```python
from build123d import *

# Parameters (mm, degrees)
SKETCH_1_R               = 2.6
EXTRUDE_1_DEPTH          = 5
EXTRUDE_2_DEPTH          = 3.5
PATTERN_CIRCULAR_4_COUNT = 3


with BuildPart() as part:
    # 草图1 → 凸台-拉伸1 (new body)
    with BuildSketch(Plane(origin=(0, 0, 0), x_dir=(1, 0, 0), z_dir=(0, 1, 0))):
        with BuildLine():
            Line((-4.913295992, -4.857418706), (-3.181245185, -3.857418706))
            ThreePointArc((-3.181245185, -3.857418706), (0, -5), (3.181245185, -3.857418706))
            Line((3.181245185, -3.857418706), (4.913295992, -4.857418706))
            Line((4.913295992, -4.857418706), (6.663295992, -1.826329793))
            Line((6.663295992, -1.826329793), (4.931245185, -0.826329793))
            ThreePointArc((4.931245185, -0.826329793), (4.330127019, 2.5), (1.75, 4.683748499))
            Line((1.75, 4.683748499), (1.75, 6.683748499))
            Line((1.75, 6.683748499), (-1.75, 6.683748499))
            Line((-1.75, 6.683748499), (-1.75, 4.683748499))
            ThreePointArc((-1.75, 4.683748499), (-4.330127019, 2.5), (-4.931245185, -0.826329793))
            Line((-4.931245185, -0.826329793), (-6.663295992, -1.826329793))
            Line((-6.663295992, -1.826329793), (-4.913295992, -4.857418706))
        make_face()
        with Locations(Location((0, 0, 0), (0, 0, 270))):
            Circle(SKETCH_1_R, mode=Mode.SUBTRACT)
    extrude(amount=EXTRUDE_1_DEPTH)

    # 草图2 → 凸台-拉伸2 (add)
    with BuildSketch(Plane(origin=(0.875, 0, 1.515544457), x_dir=(0.8660254037844383, 0, -0.5000000000000009), z_dir=(0.5000000000000008, 0, 0.8660254037844382))):
        Polygon((-4.683748499, 5), (-9.731723247, 13.632378058), (-11.731723247, 12.462833649), (-6.683748499, 3.830455591), align=None)
    extrude(amount=-EXTRUDE_2_DEPTH)


with BuildPart() as pattern_circular_4_1:
    # 阵列(圆周)4: pattern copy
    add(part.part.rotate(Axis((0, 0, 0), (0, 1, 0)), 1 * 360 / PATTERN_CIRCULAR_4_COUNT))


with BuildPart() as pattern_circular_4_2:
    # 阵列(圆周)4: pattern copy
    add(part.part.rotate(Axis((0, 0, 0), (0, 1, 0)), 2 * 360 / PATTERN_CIRCULAR_4_COUNT))


with BuildPart() as pattern_circular_4_1_1:
    add(pattern_circular_4_1.part)

    # Combine 1: read off the stored shape, not the designer's step
    # Combine 1: union 阵列(圆周)4_2, part
    add(pattern_circular_4_2.part)
    add(part.part)


solid = pattern_circular_4_1_1.part
```
Read the model definition and answer for the solid it produces. Units are mm, in the model's axes. A direction names the side the tool comes from. Give positions to 0.01 mm unless a question says otherwise; leave off trailing zeros. Order: outer loops, then holes, each group sorted by start corner. A loop starts at its lowest first (then second) coordinate and runs counter-clockwise, first axis right, second up.
(1) Find section D-D (z = -2). Give the vertices of the cut face in (x, y), plus the area to 3 significant figures.
(2) Find section A-A (x = 0). Give the vertices of the cut face in (y, z), plus the area to 3 significant figures.
(3) Given pin 1 (0.6 mm diameter, centred on y = 1.5, z = -5.5, fed in from -X); pin 2 (1.1 mm diameter, centred on x = -1, y = 2.5, fed in from -Z); pin 3 (2 mm diameter, centred on x = 0, y = 9, fed in from +Z), each flat-ended and moving along its own axis, determine where each tip first touches the part or whether it passes through.
(4) Find section B-B (z = 0). Give the vertices of the cut face in (x, y).
(5) For a pull along X with two mould halves and no side action, classify faces 1 (the flat face through (-0.025, 13.056, -10.718)), 2 (the flat face through (8.02, 8.21, 4.6)), 3 (the flat face through (-6.2, 9.26, 3.61)) as released by +X, released by -X, zero draft, split by the parting line, or undercut.
(6) Straight lines are drawn through the part: L1, parallel to X at y = 3.4, z = 0; L2, parallel to X at y = 12.25, z = -10; L3, parallel to Y at x = -2.5, z = -3.25. For each, find the intervals that lie inside material, in ascending order.
(7) For faces 4 (the flat face through (6.224, 9.256, 3.565)), 5 (the flat face through (-5.8, 1.89, 3.32)), 6 (the flat face through (-3, 5, -1)), determine the directions among +Z, -Z, +X, -X, +Y, -Y from which every point of the face is accessible in a straight line to the end or side of a thin tool.
(8) Find section C-C (y = 8). Give the vertices of the cut face in (x, z).
Result sheet:
1. outline: (-4.58, 0) - (-1.66, 0) - (-1.66, 5) - (-4.58, 5) - close; (1.66, 0) - (4.58, 0) - (4.58, 5) - (1.66, 5) - close
1. area: 29.2 mm2
2. outline: (0, -6.68) - (3.83, -6.68) - (12.46, -11.73) - (13.63, -9.73) - (5, -4.68) - (5, -2.6) - (0, -2.6) - close; (0, 2.6) - (5, 2.6) - (5, 5) - (0, 5) - close
2. area: 54.4 mm2
3. pin 1: stops at x = -1.75
3. pin 2: stops at z = -6.68
3. pin 3: stops at z = -6.44
4. outline: (-5, 0) - (-2.6, 0) - (-2.6, 5) - (-5, 5) - close; (2.6, 0) - (5, 0) - (5, 5) - (2.6, 5) - close
5. face 1: zero draft
5. face 2: released by +X
5. face 3: undercut
6. L1: x = -5 to -2.6, 2.6 to 5
6. L2: x = -1.75 to 1.75
6. L3: y = 0 to 5
7. face 4: -Z, +Y
7. face 5: +Z, -X, -Y
7. face 6: +Y
8. outline: (-8.77, 3.05) - (-6.45, 1.7) - (-4.7, 4.73) - (-7.02, 6.08) - close; (-1.75, -9.12) - (1.75, -9.12) - (1.75, -6.44) - (-1.75, -6.44) - close; (4.7, 4.73) - (6.45, 1.7) - (8.77, 3.05) - (7.02, 6.08) - close
